Autodesk Inventor part; units mm, degrees
ref_plane "YZ Plane" through (0, 0, 0) normal (1, 0, 0) x (0, 1, 0)
ref_plane "XZ Plane" through (0, 0, 0) normal (0, 1, 0) x (-1, 0, 0)
ref_plane "XY Plane" through (0, 0, 0) normal (0, 0, 1) x (1, 0, 0)
sketch "Sketch1" plane through (0, 0, 0) normal (0, 1, 0) x (-1, 0, 0)
  arc A0 (19.8614, 2.3507) -> (19.8614, -2.3507) centre (0, 0) ccw
  arc A1 (23.9872, -0.7853) -> (23.9872, 0.7853) centre (0, 0) ccw
  line L0 (0, 0) -> (20, 0) construction
  line L1 (0, 0) -> (24, 0) construction
  line L2 (23.9872, -0.7853) -> (19.8614, -2.3507)
  line L3 (23.9872, 0.7853) -> (19.8614, 2.3507)
extrude "Extrusion1" add sketch "Sketch1" along normal blind 15
pattern_circular "Circular Pattern1" count 20 over 360 about axis through (0, 0, 0) along (0, 1, 0) of "Extrusion1"
sketch "Sketch2" plane through (0, 0, 0) normal (0, -1, 0) x (1, 0, 0)
  circle A0 centre (0, 0) radius 8.6
extrude "Extrusion2" cut sketch "Sketch2" against normal blind 15
properties part number "gear_small" material "Gypsum Wall Board"
Build history of the part. All positions in model axes, mm. A direction names the side the tool comes from. Round coordinates to 2 decimals unless told otherwise and drop trailing zeros. Loops run counter-clockwise (first coordinate to the right, second up) from the corner with the lowest first, then second, coordinate; pieces in that order, holes last.
Item 1: Pin check, flat tips, straight feed: P1, Ø15.5, axis at x = 0, z = 0, coming from the +Y side; P2, Ø6, axis at x = -15.5, y = 13, coming from the +Z side; P3, Ø8, axis at x = 4.5, y = 6.5, coming from the -Z side; P4, Ø1.5, axis at y = 6.5, z = 8.5, coming from the +X side. Stop position of each tip, or through.
Item 2: Drill centre lines: line 1 along Z through (x, y) = (0, 9.25); line 2 along X through (y, z) = (3, -20.5); line 3 along Z through (x, y) = (21, 2.75). Where is each one in solid material? Low to high.
Item 3: Which spindle directions (+Z, -Z, +X, -X, +Y, -Y) get a long thin tool onto all of the face, cutting with end or side? Do faces 5 (the face through (19.756, 7.395, 3.118)), 6 (the face through (-5.303, 7.395, 21.36)), 7 (the face through (14.15, 7.395, 14.134)). Say none if no direction does.
Item 4: Saw through at B-B (z = 0). List the corners of the cut face in (x, y), then the cut area to 3 significant figures.
Item 5: Two-plate mould, pull along Z, no slides. Class faces 1 (the face through (0, 7, -24)), 2 (the face through (-17.815, 7.395, 9.09)), 3 (the face through (-20.398, 7.395, -8.265)), 4 (the face through (-11.644, 7.395, 18.676)): released by +Z, released by -Z, zero draft, split by the parting line, or undercut.
Item 6: Saw through at C-C (z = -11). List the corners of the cut face in (x, y), then the cut area to 3 significant figures.
Item 7: Saw through at A-A (x = 0). List the corners of the cut face in (y, z).
Item 8: Saw through at D-D (z = -16.5). List the corners of the cut face in (x, y).
Worked answers:
1. P1: passes through
1. P2: stops at z = 19.87
1. P3: stops at z = -23.99
1. P4: stops at x = 22.71
2. line 1: z = -24 to -8.6, 8.6 to 24
2. line 2: x = -8.26 to -4.61, -2.11 to 2.11, 4.61 to 8.26
2. line 3: z = -8.24 to -5.01, -1.92 to 1.92, 5.01 to 8.24
3. face 5: +X, +Y, -Y
3. face 6: +Z, +Y, -Y
3. face 7: +Y, -Y
4. outline: (-24, 0) - (-8.6, 0) - (-8.6, 15) - (-24, 15) - close; (8.6, 0) - (24, 0) - (24, 15) - (8.6, 15) - close
4. area: 462 mm2
5. face 1: released by -Z
5. face 2: undercut
5. face 3: undercut
5. face 4: released by +Z
6. outline: (-18.25, 0) - (18.25, 0) - (18.25, 15) - (-18.25, 15) - close
6. area: 548 mm2
7. outline: (0, -24) - (15, -24) - (15, -8.6) - (0, -8.6) - close; (0, 8.6) - (15, 8.6) - (15, 24) - (0, 24) - close
8. outline: (-14.07, 0) - (14.07, 0) - (14.07, 15) - (-14.07, 15) - close
